```python
from build123d import *

# Parameters (mm, degrees)
EXTRUDE1_DEPTH      = 9.525
EXTRUDE1_DEPTH_BACK = 9.525
SKETCH3_R           = 3.5687
EXTRUDE2_DEPTH      = 12.7
CUT_EXTRUDE1_DEPTH  = 4.7625


with BuildPart() as part:
    # Sketch1 → Extrude1 (new, two sides)
    with BuildSketch(Plane.XY) as extrude1_sk:
        with BuildLine():
            Line((-1.5875, 0), (99.695, 0))
            Line((99.695, 0), (120.3325, 20.6375))
            Line((120.3325, 20.6375), (120.3325, 50.8))
            Line((120.3325, 50.8), (109.22, 50.8))
            Line((109.22, 50.8), (109.22, 66.04))
            Line((109.22, 66.04), (79.0575, 66.04))
            Line((79.0575, 66.04), (79.0575, 50.8))
            Line((79.0575, 50.8), (45.72, 50.8))
            ThreePointArc((45.72, 50.8), (38.535795103, 47.824204897), (35.56, 40.64))
            Line((35.56, 40.64), (30.1625, 40.64))
            ThreePointArc((30.1625, 40.64), (26.794903955, 39.245096045), (25.4, 35.8775))
            Line((25.4, 35.8775), (25.4, 35.56))
            Line((25.4, 35.56), (9.8425, 35.56))
            ThreePointArc((9.8425, 35.56), (6.474903955, 34.165096045), (5.08, 30.7975))
            Line((5.08, 30.7975), (5.08, 27.94))
            Line((5.08, 27.94), (0, 27.94))
            Line((0, 27.94), (0, 13.49375))
            Line((0, 13.49375), (-4.7625, 13.49375))
            Line((-4.7625, 13.49375), (-4.7625, 3.175))
            ThreePointArc((-4.7625, 3.175), (-3.83256403, 0.92993597), (-1.5875, 0))
        make_face()
    extrude(amount=EXTRUDE1_DEPTH)
    extrude(extrude1_sk.sketch, amount=-EXTRUDE1_DEPTH_BACK)


with BuildPart() as body_2:
    # Sketch3 → Extrude2 (new body)
    with BuildSketch(Plane.ZY):
        with Locations((0, 20.6502)):
            Circle(SKETCH3_R)
    extrude(amount=-EXTRUDE2_DEPTH)


with BuildPart() as part_1:
    add(part.part)

    # Combine1: cut body 2
    add(body_2.part, mode=Mode.SUBTRACT)

    # Sketch4 → Cut-Extrude1 (cut)
    with BuildSketch(Plane.ZY.offset(4.7625)):
        Polygon((-9.525, 20.0025), (-9.525, 0), (-5.55625, 0), (-5.55625, 16.03375), align=None)
        Polygon((5.55625, 0), (9.525, 0), (9.525, 20.0025), (5.55625, 16.03375), align=None)
    extrude(amount=-CUT_EXTRUDE1_DEPTH, mode=Mode.SUBTRACT)


solid = part_1.part
```
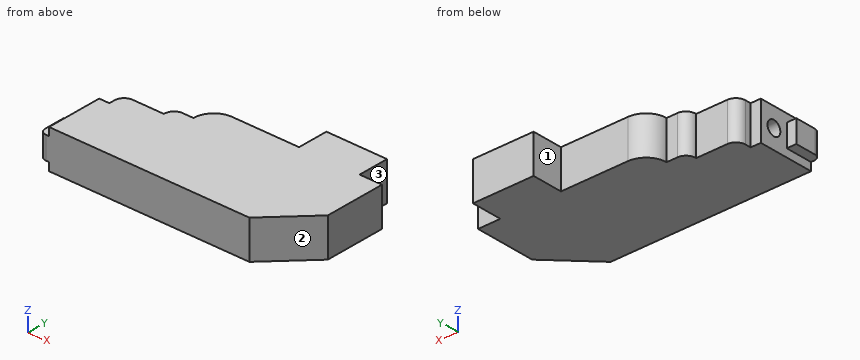
Work out the finished part from the listing and answer in its coordinate system (mm). Face numbers are marked on the shaded views. A direction names the side the tool comes from. Give positions to 0.01 mm unless a question says otherwise; leave off trailing zeros. Loops run counter-clockwise (first coordinate to the right, second up) from the corner with the lowest first, then second, coordinate; pieces in that order, holes last. Notation, with made-up numbers: (-22.75, 69) - (16.25, 69) arc R15 ccw to (16.25, 95) - close; hole circle Ø2 at (-35, 75). An arc over 180 degrees is marked (long way). Use CSV: the item, a comma, the result in double quotes. Start each with the question number.
(1) Each of these flat-tipped pins is pushed along its axis until it touches: pin 1 (8 mm diameter, centred on x = 56.5, z = 5, fed in from +Y); pin 2 (1.5 mm diameter, centred on y = 18.5, z = 1, fed in from +X) (3 decimals); pin 3 (4.5 mm diameter, centred on y = 62, z = -2, fed in from -X); pin 4 (5 mm diameter, centred on y = 15, z = -4.5, fed in from -X). Where does it stop, or does it pass through?
(2) Find section B-B, the plane x = 15.5. Determine the outline of the cut face in (y, z) (3 decimals).
(3) Find section C-C, the plane y = 52. Determine the outline of the cut face in (x, z) (1 decimal).
(4) Find the intervals of material crossed by L1, parallel to X at y = 21.5, z = 7.5; L2, parallel to X at y = 60, z = 8; L3, parallel to Y at x = 18, z = -3.75, in increasing order.
(5) A tool of negligible diameter and unlimited length cuts with its end or side. For the marked faces 1, 2 and 3, from which of +Z, -Z, +X, -X, +Y, -Y can it reach the whole face along a straight path? Write none if from no direction.
Results found:
1,pin 1,"y = 50.8"
1,pin 2,"x = 118.945"
1,pin 3,"x = 79.06"
1,pin 4,"x = -4.76"
2,outline,"(0, -9.525) - (35.56, -9.525) - (35.56, 9.525) - (0, 9.525) - close"
3,outline,"(79.1, -9.5) - (109.2, -9.5) - (109.2, 9.5) - (79.1, 9.5) - close"
4,L1,"0 to 120.33"
4,L2,"79.06 to 109.22"
4,L3,"0 to 35.56"
5,face 1,"+Z, -Z, -X, +Y"
5,face 2,"+Z, -Z, +X, -Y"
5,face 3,"+Z, -Z, +X, +Y"
